```python
from build123d import *

# Parameters (mm, degrees)
SKETCH1_W               = 36.5125
SKETCH1_H               = 6.35
CUT_EXTRUDE1_DEPTH      = 53.025453506
CUT_EXTRUDE1_DEPTH_BACK = 53.025453506
SKETCH2_R               = 11.8745
SKETCH2_R_2             = 3.175
SKETCH2_R_3             = 4.1275
CUT_EXTRUDE2_DEPTH      = 53.025453506
CUT_EXTRUDE2_DEPTH_BACK = 53.025453506
SKETCH3_R               = 3.175


with BuildPart() as part:
    # Sketch1 → Revolve1 (revolve)
    with BuildSketch(Plane.XY, mode=Mode.PRIVATE) as revolve1_sk:
        with Locations((18.25625, 3.175)):
            Rectangle(SKETCH1_W, SKETCH1_H)
    revolve(revolve1_sk.sketch.rotate(Axis((0, 0, 0), (0, 1, 0)), 90), axis=Axis((0, 0, 0), (0, 1, 0)))

    # Sketch2 → Cut-Extrude1 (cut, two sides: drawn at the far end of the back side and taken through both)
    with BuildSketch(Plane(origin=(0, 6.35, 0), x_dir=(1, 0, 0), z_dir=(0, 1, 0)).offset(-CUT_EXTRUDE1_DEPTH_BACK)):
        with Locations(Location((-12.7, 15.699275429, 0), (0, 0, 270))):
            Circle(SKETCH2_R)
        with Locations(Location((12.7, 15.699275429, 0), (0, 0, 270))):
            Circle(SKETCH2_R)
        with Locations(Location((0, 25.859275429, 0), (0, 0, 270))):
            Circle(SKETCH2_R_2)
        with Locations(Location((0, 5.539275429, 0), (0, 0, 270))):
            Circle(SKETCH2_R_2)
        with Locations(Location((0, -14.605, 0), (0, 0, 270))):
            Circle(SKETCH2_R_3)
    extrude(amount=CUT_EXTRUDE1_DEPTH + CUT_EXTRUDE1_DEPTH_BACK, mode=Mode.SUBTRACT)

    # Sketch3 → Cut-Extrude2 (cut, two sides: drawn at the far end of the back side and taken through both)
    with BuildSketch(Plane(origin=(0, 6.35, 0), x_dir=(1, 0, 0), z_dir=(0, 1, 0)).offset(-CUT_EXTRUDE2_DEPTH_BACK)):
        with Locations(Location((-25.4, -1.905, 0), (0, 0, 270))):
            Circle(SKETCH3_R)
        with Locations(Location((25.4, -1.905, 0), (0, 0, 270))):
            Circle(SKETCH3_R)
    extrude(amount=CUT_EXTRUDE2_DEPTH + CUT_EXTRUDE2_DEPTH_BACK, mode=Mode.SUBTRACT)


solid = part.part
```
Source: CAD feature listing. Evaluate the final solid. Frame: model axes, mm. Round coordinates to 2 decimals unless told otherwise and drop trailing zeros. Loops run counter-clockwise (first coordinate to the right, second up) from the corner with the lowest first, then second, coordinate; pieces in that order, holes last.
1. Section query B-B on x = -14.5. Output: boundary loops of the cut face in (y, z).
2. Ray query, L1, parallel to X at y = 1.5, z = -19; L2, parallel to X at y = 5.5, z = -7; L3, parallel to X at y = 5.5, z = -17. Return the intervals inside material, ascending.
3. Contact query for flat-ended pins moving along their axis: pin 1 (3 mm diameter, centred on x = 21.5, y = 1, fed in from +Z); pin 2 (7.5 mm diameter, centred on x = 0, z = -25.86, fed in from -Y); pin 3 (1.5 mm diameter, centred on y = 4.5, z = 8.5, fed in from +X); pin 4 (1.5 mm diameter, centred on x = 9, y = 3.5, fed in from +Z). Output: stop coordinate, or through.
4. Section query C-C on y = 3. Give the number of separate pieces and of enclosed holes in the cut face, and give its area (3 significant figures).
5. Mould query, pull axis Z, two halves, no side actions, for faces 1 (the flat face through (-1, 0, 8)), 2 (the cylindrical face through (-1.93, 3.13, -8.06)), 3 (the cylindrical face through (32.39, 3.22, -16.85)). Classes: released by +Z, released by -Z, zero draft, split by the parting line, or undercut.
6. Section query D-D on z = 15. Output: boundary loops of the cut face in (x, y).
7. Section query A-A on z = 0. Output: boundary loops of the cut face in (x, y), and give its area (3 significant figures).
Answers below:
1. outline: (0, -33.51) - (6.35, -33.51) - (6.35, -27.44) - (0, -27.44) - close; (0, -3.96) - (6.35, -3.96) - (6.35, 33.51) - (0, 33.51) - close
2. L1: x = -31.18 to -24.11, -1.29 to 1.29, 24.11 to 31.18
2. L2: x = -35.84 to -20.78, -4.62 to -2.82, 2.82 to 4.62, 20.78 to 35.84
2. L3: x = -32.31 to -24.5, -0.9 to 0.9, 24.5 to 32.31
3. pin 1: stops at z = 30.55
3. pin 2: stops at y = 0
3. pin 3: stops at x = 35.68
3. pin 4: stops at z = 35.57
4. separate pieces: 1
4. enclosed holes: 7
4. area: 3,120 mm2
5. face 1: zero draft
5. face 2: undercut
5. face 3: split by the parting line
6. outline: (-33.29, 0) - (-4.11, 0) - (-4.11, 6.35) - (-33.29, 6.35) - close; (4.11, 0) - (33.29, 0) - (33.29, 6.35) - (4.11, 6.35) - close
7. outline: (-36.51, 0) - (-27.94, 0) - (-27.94, 6.35) - (-36.51, 6.35) - close; (-22.86, 0) - (22.86, 0) - (22.86, 6.35) - (-22.86, 6.35) - close; (27.94, 0) - (36.51, 0) - (36.51, 6.35) - (27.94, 6.35) - close
7. area: 399 mm2
